```python
from build123d import *

# Parameters (mm, degrees)
SKETCH_1_R               = 37
SKETCH_1_R_2             = 2
SKETCH_1_R_3             = 27
EXTRUDE_1_DEPTH          = 3
SKETCH_2_R               = 90
SKETCH_2_R_2             = 20
SKETCH_2_R_3             = 42
EXTRUDE_2_DEPTH          = 3
EXTRUDE_3_DEPTH          = 3
CUT_EXTRUDE_1_DEPTH      = 128.314571044
CUT_EXTRUDE_1_DEPTH_BACK = 128.314571044
SKETCH_5_R               = 20
CUT_EXTRUDE_2_DEPTH      = 128.314571044
CUT_EXTRUDE_2_DEPTH_BACK = 128.314571044


with BuildPart() as part:
    # Sketch 1 → Extrude 1 (new body)
    with BuildSketch(Plane.XY):
        Circle(SKETCH_1_R)
        with Locations((-32, 0)):
            Circle(SKETCH_1_R_2, mode=Mode.SUBTRACT)
        with Locations((0, 32)):
            Circle(SKETCH_1_R_2, mode=Mode.SUBTRACT)
        with Locations((32, 0)):
            Circle(SKETCH_1_R_2, mode=Mode.SUBTRACT)
        with Locations((0, -32)):
            Circle(SKETCH_1_R_2, mode=Mode.SUBTRACT)
        Circle(SKETCH_1_R_3, mode=Mode.SUBTRACT)
    extrude(amount=EXTRUDE_1_DEPTH)



with BuildPart() as body_2:
    # Sketch 2 → Extrude 2 (new body)
    with BuildSketch(Plane.XY.offset(3)):
        Circle(SKETCH_2_R)
        with Locations((-63.751104535, -17.082056977)):
            Circle(SKETCH_2_R_2, mode=Mode.SUBTRACT)
        with Locations((-17.082056977, 63.751104535)):
            Circle(SKETCH_2_R_2, mode=Mode.SUBTRACT)
        with Locations((63.751104535, 17.082056977)):
            Circle(SKETCH_2_R_2, mode=Mode.SUBTRACT)
        with Locations((17.082056977, -63.751104535)):
            Circle(SKETCH_2_R_2, mode=Mode.SUBTRACT)
        Circle(SKETCH_2_R_3, mode=Mode.SUBTRACT)
    extrude(amount=-EXTRUDE_2_DEPTH)


with BuildPart() as part_1:
    add(part.part)

    add(body_2.part)  # Extrude 3 merges body 2
    # Sketch 3 → Extrude 3 (add)
    with BuildSketch(Plane.XY.offset(3)):
        Polygon((-41.892720131, 3), (-34.060564973, 3), (-34.060564973, -3), (-43.204810996, -3), (-43.204810996, 3), align=None)
        Polygon((-28.429094491, 32.671735178), (-27.501306144, 31.743946831), (-21.96313612, 26.205776807), (-26.205776807, 21.96313612), (-32.671735178, 28.429094491), align=None)
        Polygon((3, 43.204810996), (3, 41.892720131), (3, 34.060564973), (-3, 34.060564973), (-3, 43.204810996), align=None)
        Polygon((32.671735178, 28.429094491), (31.743946831, 27.501306144), (26.205776807, 21.96313612), (21.96313612, 26.205776807), (28.429094491, 32.671735178), align=None)
        Polygon((43.204810996, -3), (41.892720131, -3), (34.060564973, -3), (34.060564973, 3), (43.204810996, 3), align=None)
        Polygon((28.429094491, -32.671735178), (27.501306144, -31.743946831), (21.96313612, -26.205776807), (26.205776807, -21.96313612), (32.671735178, -28.429094491), align=None)
        Polygon((-3, -43.204810996), (-3, -41.892720131), (-3, -34.060564973), (3, -34.060564973), (3, -43.204810996), align=None)
        Polygon((-32.671735178, -28.429094491), (-31.743946831, -27.501306144), (-26.205776807, -21.96313612), (-21.96313612, -26.205776807), (-28.429094491, -32.671735178), align=None)
    extrude(amount=-EXTRUDE_3_DEPTH)

    # Sketch 5 → Cut-Extrude 1 (cut, two sides: drawn at the far end of the back side and taken through both)
    with BuildSketch(Plane.XY.offset(3).offset(-CUT_EXTRUDE_1_DEPTH_BACK)):
        with Locations((-57.15767665, 33)):
            Circle(SKETCH_5_R)
        with Locations((33, 57.15767665)):
            Circle(SKETCH_5_R)
        with Locations((57.15767665, -33)):
            Circle(SKETCH_5_R)
        with Locations((-33, -57.15767665)):
            Circle(SKETCH_5_R)
    extrude(amount=CUT_EXTRUDE_1_DEPTH + CUT_EXTRUDE_1_DEPTH_BACK, mode=Mode.SUBTRACT)

    # Sketch 6 → Cut-Extrude 2 (cut, two sides: drawn at the far end of the back side and taken through both)
    with BuildSketch(Plane(origin=(0, 0, 0), x_dir=(1, 0, 0), z_dir=(0, 1, 0)).offset(-CUT_EXTRUDE_2_DEPTH_BACK)):
        Polygon((100.374072396, 28.225781081), (-90, 7.369193783), (-90, 0), (-90, -1.2), (96.19546412, -1.2), align=None)
    extrude(amount=CUT_EXTRUDE_2_DEPTH + CUT_EXTRUDE_2_DEPTH_BACK, mode=Mode.SUBTRACT)


solid = part_1.part
```
Read the model definition and answer for the solid it produces. Units are mm, in the model's axes. Coordinates: 2 decimals unless noted, no trailing zeros. Loops run counter-clockwise (first coordinate to the right, second up) from the corner with the lowest first, then second, coordinate; pieces in that order, holes last.
(1) The mould has two halves that part along X. Classify faces 1 (the face through (41.53, -79.845, 2.113)), 2 (the face through (-5.85, -26.36, 2.09)): released by +X, released by -X, zero draft, split by the parting line, or undercut.
Solution:
face 1: split by the parting line
face 2: undercut
(2) Flat-ended cylindrical pins translate along their axes: pin 1 Ø2.5 at (x, y) = (0, -32) entering from +Z; pin 2 Ø0.9 at (y, z) = (-40, 2.5) entering from +X; pin 3 Ø0.9 at (x, z) = (40, 2) entering from +Y; pin 4 Ø0.5 at (y, z) = (40.5, 2) entering from -X. Find the tip coordinate at first contact, or state that the pin passes through.
Solution:
pin 1: passes through
pin 2: stops at x = 80.84
pin 3: stops at y = 80.84
pin 4: stops at x = -80.5
(3) The part is cut by section C-C (z = 2.55). Count the separate pieces of the cut face and the enclosed holes in it, and give its area (3 significant figures).
Solution:
separate pieces: 1
enclosed holes: 21
area: 12,100 mm2
(4) The part is cut by section B-B (x = 21.5). Determine the outline of the cut face in (y, z).
Solution:
outline: (-87.39, 1.2) - (-83.26, 1.2) - (-83.26, 3) - (-87.39, 3) - close; (-44.25, 1.2) - (-36.08, 1.2) - (-36.08, 3) - (-44.25, 3) - close; (-30.11, 1.2) - (-16.33, 1.2) - (-16.33, 3) - (-30.11, 3) - close; (16.33, 1.2) - (30.11, 1.2) - (30.11, 3) - (16.33, 3) - close; (36.08, 1.2) - (40.79, 1.2) - (40.79, 3) - (36.08, 3) - close; (73.52, 1.2) - (87.39, 1.2) - (87.39, 3) - (73.52, 3) - close
(5) Consider line 1 along X through (y, z) = (-6.5, 2.6); line 2 along Y through (x, z) = (-5.5, 1.55); line 3 along X through (y, z) = (-59.5, 1.5). Determine where each line is inside the solid, lowest interval first.
Solution:
line 1: x = -89.76 to -80.72, -46.78 to -41.49, -36.42 to -26.21, 26.21 to 36.42, 41.49 to 89.76
line 2: y = -89.83 to -41.64, -36.59 to -26.43, 26.43 to 36.59, 41.64 to 47.45, 80.06 to 89.83
line 3: x = -67.53 to -52.86, -13.14 to -2.46, 36.63 to 67.53
(6) The part is cut by section A-A (x = 50). Determine the outline of the cut face in (y, z), and give its area (3 significant figures).
Solution:
outline: (-74.83, 1.2) - (-51.68, 1.2) - (-51.68, 3) - (-74.83, 3) - close; (-14.32, 1.2) - (2.56, 1.2) - (2.56, 3) - (-14.32, 3) - close; (31.6, 1.2) - (46.62, 1.2) - (46.62, 3) - (31.6, 3) - close; (67.69, 1.2) - (74.83, 1.2) - (74.83, 3) - (67.69, 3) - close
area: 112 mm2
